Check sheet for the modelled part. Datum: model origin and axes. Units: mm. A direction names the side the tool comes from. Coordinates: 2 decimals unless noted, no trailing zeros. Loops run counter-clockwise (first coordinate to the right, second up) from the corner with the lowest first, then second, coordinate; pieces in that order, holes last. Notation, with made-up numbers: M 11.25,76 L 22.25,76 A18 ccw 22.25,94 Z; hole C 79,34 d8. An arc over 180 degrees is marked long. Return JSON: item names as keys, results as strings.
from build123d import *

# Parameters (mm, degrees)
SKETCH1_R           = 24.5
BOSS_EXTRUDE1_DEPTH = 5.5
SKETCH2_R           = 2.5
CUT_EXTRUDE1_DEPTH  = 6.6
SKETCH6_R           = 2.5
BOSS_EXTRUDE2_DEPTH = 2.5
FILLET1_R           = 0.5


with BuildPart() as part:
    # Sketch1 → Boss-Extrude1 (new body)
    with BuildSketch(Plane(origin=(0, 0, 0), x_dir=(1, 0, 0), z_dir=(0, 1, 0))):
        with Locations(Location((0, 0, 0), (0, 0, 270))):
            Circle(SKETCH1_R)
    extrude(amount=BOSS_EXTRUDE1_DEPTH)

    # Sketch2 → Cut-Extrude1 (cut)
    with BuildSketch(Plane(origin=(0, 5.5, 0), x_dir=(1, 0, 0), z_dir=(0, 1, 0))):
        with Locations(Location((-9, -15.588457268, 0), (0, 0, 270))):
            Circle(SKETCH2_R)
        with Locations(Location((-15.588457268, 9, 0), (0, 0, 270))):
            Circle(SKETCH2_R)
        with Locations(Location((-18, 0, 0), (0, 0, 270))):
            Circle(SKETCH2_R)
        with Locations(Location((0, -18, 0), (0, 0, 270))):
            Circle(SKETCH2_R)
        with Locations(Location((9, -15.588457268, 0), (0, 0, 270))):
            Circle(SKETCH2_R)
        with Locations(Location((-9, 15.588457268, 0), (0, 0, 270))):
            Circle(SKETCH2_R)
        with Locations(Location((9, 15.588457268, 0), (0, 0, 270))):
            Circle(SKETCH2_R)
        with Locations(Location((15.588457268, 9, 0), (0, 0, 270))):
            Circle(SKETCH2_R)
        with Locations(Location((18, 0, 0), (0, 0, 270))):
            Circle(SKETCH2_R)
    extrude(amount=-CUT_EXTRUDE1_DEPTH, mode=Mode.SUBTRACT)

    # Sketch6 → Boss-Extrude2 (add)
    with BuildSketch(Plane(origin=(0, 5.5, 0), x_dir=(1, 0, 0), z_dir=(0, 1, 0))):
        with Locations(Location((0, 15.9, 0), (0, 0, 270))):
            Circle(SKETCH6_R)
        with Locations(Location((13.76980392, -7.95, 0), (0, 0, 270))):
            Circle(SKETCH6_R)
        with Locations(Location((-13.76980392, -7.95, 0), (0, 0, 270))):
            Circle(SKETCH6_R)
    extrude(amount=BOSS_EXTRUDE2_DEPTH)

    # Fillet1
    fillet1_edges = [part.edges().sort_by_distance(p)[0] for p in [
        (0, 8, -18.4),
        (13.76980392, 8, 5.45),
        (-13.76980392, 8, 5.45),
    ]]
    fillet(fillet1_edges, radius=FILLET1_R)


solid = part.part
1) Section check C-C on y = 3.25. Count the separate pieces of the cut face and the enclosed holes in it, then the cut area to 3 significant figures.
Answers:
{"separate pieces": "1", "enclosed holes": "9", "area": "1,710 mm²"}
2) Section check D-D on x = -10. Record the cut outline in (y, z), then the cut area to 3 significant figures.
Answers:
{"outline": "M 0,-22.37 L 5.5,-22.37 L 5.5,-17.88 L 0,-17.88 Z; M 0,-13.3 L 5.5,-13.3 L 5.5,13.3 L 0,13.3 Z; M 0,17.88 L 5.5,17.88 L 5.5,22.37 L 0,22.37 Z", "area": "196 mm²"}
3) Set-up check for faces 1 (the face through (6.56, 2.79, 15.05)), 2 (the face through (1.69, 6.49, -17.74)): record each of +Z, -Z, +X, -X, +Y, -Y from which the full face is reachable in a straight line by a thin tool's end or side.
Answers:
{"face 1": "+Y, -Y", "face 2": "+Y"}
4) Go/stop test with a flat-tipped pin: pin 1 Ø8 at (x, z) = (11, -11) entering from +Y. Record where the tip stops, or that it passes through.
Answers:
{"pin 1": "y = 5.5"}
5) Draft check along Z on faces 3 (the face through (0, 5.5, 0)), 4 (the face through (-15.52, 2.79, -0.33)), 5 (the face through (-14.73, 6.49, 10.26)). Enter one of: +Z half, -Z half, draft (parallel to the pull), parting line (faces both ways), or undercut.
Answers:
{"face 3": "draft", "face 4": "undercut", "face 5": "parting line"}
6) Scan lines: line 1 along X through (y, z) = (2.8, 0); line 2 along X through (y, z) = (1.25, -9); line 3 along X through (y, z) = (2, 16.5). Record each from-to range of solid material in increasing order. Write a range as [from, to].
Answers:
{"line 1": "[-24.5, -20.5], [-15.5, 15.5], [20.5, 24.5]", "line 2": "[-22.79, -18.09], [-13.09, 13.09], [18.09, 22.79]", "line 3": "[-18.11, -11.33], [-6.67, -2], [2, 6.67], [11.33, 18.11]"}
7) Section check B-B on x = 0. Record the cut outline in (y, z).
Answers:
{"outline": "M 0,-24.5 L 5.5,-24.5 L 5.5,-18.4 L 7.5,-18.4 A0.5 ccw 8,-17.9 L 8,-13.9 A0.5 ccw 7.5,-13.4 L 5.5,-13.4 L 5.5,15.5 L 0,15.5 Z; M 0,20.5 L 5.5,20.5 L 5.5,24.5 L 0,24.5 Z"}
8) Section check A-A on z = 0. Record the cut outline in (x, y), then the cut area to 4 significant figures.
Answers:
{"outline": "M -24.5,0 L -20.5,0 L -20.5,5.5 L -24.5,5.5 Z; M -15.5,0 L 15.5,0 L 15.5,5.5 L -15.5,5.5 Z; M 20.5,0 L 24.5,0 L 24.5,5.5 L 20.5,5.5 Z", "area": "214.5 mm²"}
